Source: CAD feature listing. Evaluate the final solid. Frame: model axes, mm. Round coordinates to 2 decimals unless told otherwise and drop trailing zeros. Write each loop counter-clockwise with the first axis right and the second up, starting at its lowest first coordinate (ties: lowest second). Pieces come first, ordered by that corner, then holes. Notation, with made-up numbers: M -1.5,57.5 L 53.5,57.5 A28 cw 53.5,79.5 Z; hole C 53.5,-39.5 d1. An arc over 180 degrees is marked long. Answer in a Markdown table with one row per item.
from build123d import *

# Parameters (mm, degrees)
SKETCH1_R           = 6.35
SKETCH1_R_2         = 4.7625
BOSS_EXTRUDE1_DEPTH = 6.35


with BuildPart() as part:
    # Sketch1 → Boss-Extrude1 (new body)
    with BuildSketch(Plane(origin=(0, 0, 0), x_dir=(1, 0, 0), z_dir=(0, 1, 0))):
        Polygon((0, -86.324674442), (0, -139.7), (71.282950652, -139.7), (304.8, -86.324674442), (304.8, 86.324674442), (71.282950652, 139.7), (0, 139.7), (0, 86.324674442), (0, 6.35), (0, -6.35), align=None)
        with Locations(Location((41.27321438, -127, 0), (0, 0, 270))):
            Circle(SKETCH1_R, mode=Mode.SUBTRACT)
        with Locations(Location((41.27321438, 127, 0), (0, 0, 90))):
            Circle(SKETCH1_R, mode=Mode.SUBTRACT)
        with Locations(Location((6.34821438, 0, 0), (0, 0, 270))):
            Circle(SKETCH1_R_2, mode=Mode.SUBTRACT)
        Polygon((279.4, 25.4), (279.4, -25.4), (25.4, -25.4), (25.4, -6.35), (25.4, 6.35), (25.4, 25.4), align=None, mode=Mode.SUBTRACT)
    extrude(amount=BOSS_EXTRUDE1_DEPTH)


solid = part.part
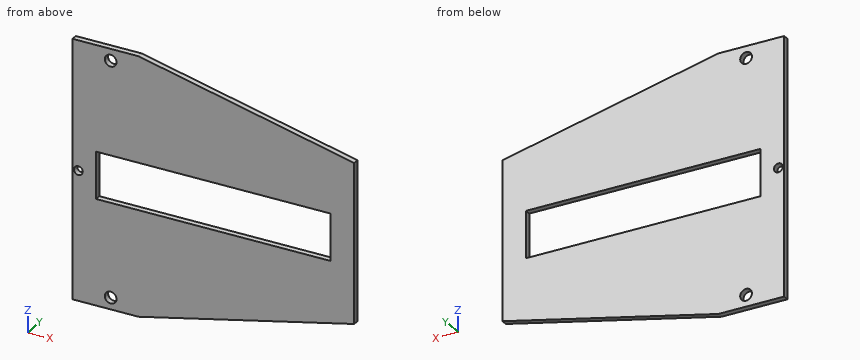
Q1. Contact query for flat-ended pins moving along their axis: pin 1 Ø3 at (x, y) = (151.5, 4.5) entering from -Z; pin 2 Ø3 at (x, y) = (108.5, 2.5) entering from -Z; pin 3 Ø1 at (x, y) = (252, 2.5) entering from -Z. Output: stop coordinate, or through.
Solutions:
| item | result |
|---|---|
| pin 1 | stops at z = -121.71 |
| pin 2 | stops at z = -131.54 |
| pin 3 | stops at z = -98.51 |
Q2. Section C-C (z = 127). Return loops of the section in (x, y).
Solutions:
| item | result |
|---|---|
| outline | M 0,0 L 34.92,0 L 34.92,6.35 L 0,6.35 Z; M 47.62,0 L 126.85,0 L 126.85,6.35 L 47.62,6.35 Z |
Q3. Section B-B (x = 189). Return loops of the section in (y, z).
Solutions:
| item | result |
|---|---|
| outline | M 0,-112.79 L 6.35,-112.79 L 6.35,-25.4 L 0,-25.4 Z; M 0,25.4 L 6.35,25.4 L 6.35,112.79 L 0,112.79 Z |
Q4. Material intervals for probe 1 along X at (y, z) = (4.75, 0); probe 2 along Z at (x, y) = (65, 1.25); probe 3 along X at (y, z) = (1.5, 12), sorted ascending.
Solutions:
| item | result |
|---|---|
| probe 1 | x = 0 to 1.59, 11.11 to 25.4, 279.4 to 304.8 |
| probe 2 | z = -139.7 to -25.4, 25.4 to 139.7 |
| probe 3 | x = 0 to 25.4, 279.4 to 304.8 |
Q5. Section A-A (z = 0). Return loops of the section in (x, y), and give its area (3 significant figures).
Solutions:
| item | result |
|---|---|
| outline | M 0,0 L 1.59,0 L 1.59,6.35 L 0,6.35 Z; M 11.11,0 L 25.4,0 L 25.4,6.35 L 11.11,6.35 Z; M 279.4,0 L 304.8,0 L 304.8,6.35 L 279.4,6.35 Z |
| area | 262 mm2 |
Q6. Section D-D (y = 1.75). State how many separate pieces and enclosed holes the cut face has, and give its area (3 significant figures).
Solutions:
| item | result |
|---|---|
| separate pieces | 1 |
| enclosed holes | 4 |
| area | 59,500 mm2 |
